Design review of the part built by this model. Coordinates are the model's own, in mm. A direction names the side the tool comes from. Round coordinates to 2 decimals unless told otherwise and drop trailing zeros. Order: outer loops, then holes, each group sorted by start corner. A loop starts at its lowest first (then second) coordinate and runs counter-clockwise, first axis right, second up.
from build123d import *

# Parameters (mm, degrees)
EXTRUDE1_DEPTH     = 254
SKETCH2_R          = 1.5875
EXTRUDE2_DEPTH     = 1.5875
SKETCH3_R          = 1.5875
CUT_EXTRUDE3_DEPTH = 255.634208228
SKETCH5_W          = 11.1125
SKETCH5_H          = 12.7
CUT_EXTRUDE4_DEPTH = 1.5875
SKETCH6_R          = 1.5875
CUT_EXTRUDE5_DEPTH = 1.5875
SKETCH7_R          = 1.5875
CUT_EXTRUDE6_DEPTH = 1.5875


with BuildPart() as part:
    # Sketch1 → Extrude1 (new body)
    with BuildSketch(Plane.XY):
        Polygon((0, 0), (0, 12.7), (-1.5875, 12.7), (-1.5875, 1.5875), (-12.7, 1.5875), (-12.7, 0), align=None)
    extrude(amount=EXTRUDE1_DEPTH)

    # Sketch2 → Extrude2 (cut)
    with BuildSketch(Plane(origin=(0, 0, 0), x_dir=(0, 0, -1), z_dir=(1, 0, 0))):
        with Locations((-247.65, 6.35)):
            Circle(SKETCH2_R)
        with Locations((-184.15, 6.35)):
            Circle(SKETCH2_R)
    extrude(amount=-EXTRUDE2_DEPTH, mode=Mode.SUBTRACT)

    # Sketch3 → Cut-Extrude3 (cut, through all)
    with BuildSketch(Plane(origin=(0, 0, 0), x_dir=(0, 0, -1), z_dir=(1, 0, 0))):
        with Locations((-24.310512242, 6.35)):
            Circle(SKETCH3_R)
        with Locations((-14.207724106, 6.35)):
            Circle(SKETCH3_R)
    extrude(amount=-CUT_EXTRUDE3_DEPTH, mode=Mode.SUBTRACT)

    # Sketch5 → Cut-Extrude4 (cut)
    with BuildSketch(Plane(origin=(0, 1.5875, 0), x_dir=(1, 0, 0), z_dir=(0, 1, 0))):
        with Locations((-7.14375, -6.35)):
            Rectangle(SKETCH5_W, SKETCH5_H)
    extrude(amount=-CUT_EXTRUDE4_DEPTH, mode=Mode.SUBTRACT)

    # Sketch6 → Cut-Extrude5 (cut)
    with BuildSketch(Plane(origin=(0, 0, 0), x_dir=(0, 0, -1), z_dir=(1, 0, 0))):
        with Locations((-6.35, 12.7)):
            Circle(SKETCH6_R)
        with Locations((-6.35, 0)):
            Circle(SKETCH6_R)
    extrude(amount=-CUT_EXTRUDE5_DEPTH, mode=Mode.SUBTRACT)

    # Sketch7 → Cut-Extrude6 (cut)
    with BuildSketch(Plane(origin=(0, 0, 0), x_dir=(0, 0, -1), z_dir=(1, 0, 0))):
        with Locations((-34.413300378, 6.35)):
            Circle(SKETCH7_R)
    extrude(amount=-CUT_EXTRUDE6_DEPTH, mode=Mode.SUBTRACT)


solid = part.part
1) To check wall thickness, follow line 1 along Y through (x, z) = (-0.55, 184.15); line 2 along Y through (x, z) = (-3, 228); line 3 along X through (y, z) = (2.5, 33.5). State the ranges of each line that lie inside material, in increasing order.
Results:
line 1: y = 0 to 4.76, 7.94 to 12.7
line 2: y = 0 to 1.59
line 3: x = -1.59 to 0
2) Take a section at B-B on x = -8.25. Give the boundary of the cut face in (y, z).
Results:
outline: (0, 12.7) - (1.59, 12.7) - (1.59, 254) - (0, 254) - close
3) Take a section at A-A on z = 85.5. Give the boundary of the cut face in (x, y).
Results:
outline: (-12.7, 0) - (0, 0) - (0, 12.7) - (-1.59, 12.7) - (-1.59, 1.59) - (-12.7, 1.59) - close
4) Clearance check with flat-ended pins moving along their axes: P1, Ø4, axis at x = -6, y = 2, coming from the -Z side; P2, Ø3.5, axis at y = 6.35, z = 184.15, coming from the -X side; P3, Ø4, axis at x = -7.5, z = 49.5, coming from the +Y side. State where each tip first meets the part, or that it passes through.
Results:
P1: stops at z = 12.7
P2: stops at x = -1.59
P3: stops at y = 1.59
5) For faces 1 (the face through (-4, 1, 254)), 2 (the face through (-7, 1.588, 132)), list the 3-axis set-ups (+Z, -Z, +X, -X, +Y, -Y) from which the entire face can be reached by the end or side of a thin tool; tool diameter is ignored.
Results:
face 1: +Z, +X, -X, +Y, -Y
face 2: +Z, -Z, -X, +Y
